Could you check a few things on this model? Use its own coordinates, in mm. Face numbers are marked on the shaded views. A direction names the side the tool comes from. Round coordinates to 2 decimals unless told otherwise and drop trailing zeros. Write each loop counter-clockwise with the first axis right and the second up, starting at its lowest first coordinate (ties: lowest second). Pieces come first, ordered by that corner, then holes. Notation, with made-up numbers: (62, 60.25) - (114, 60.25) arc R17 ccw to (114, 79.25) - close; hole circle Ø7 at (6.5, -9.5). An arc over 180 degrees is marked (long way). Write each question's results on one line, items separated by ' | '. Start each with the question number.
(1) Imagine slicing it at D-D on z = 0.75. Write out the boundary of the cut face in (x, y).
(2) Imagine slicing it at C-C on z = 5. Write out the boundary of the cut face in (x, y).
(3) Imagine slicing it at B-B on y = 3.4. Write out the boundary of the cut face in (x, z).
(4) Imagine slicing it at A-A on x = 8. Write out the boundary of the cut face in (y, z), then the cut area to 3 significant figures.
(5) On a 3-axis mill with a long thin cutter (end or side, diameter ignored), from which of +Z, -Z, +X, -X, +Y, -Y can I reach the whole of each face in a straight line? I mean the marked faces 1, 2 and 3. Say none if no direction works.
(6) For P1, Ø0.9, axis at x = -24, y = 2, coming from the +Z side; P2, Ø2.5, axis at x = -31, y = 1.5, coming from the +Z side; P3, Ø3, axis at y = 2.5, z = 4, coming from the -X side, each with a flat end and sliding along its axis, tell me the tip position at first contact or that it passes through.
(7) Please list where these lines run through material, in increasing order: line 1 (X direction, y = 2, z = 0); line 2 (Z direction, x = 11.5, y = 3.5); line 3 (Y direction, x = -24, z = 3.9). Write a range as [from, to].
```python
from build123d import *

# Parameters (mm, degrees)
SKETCH1_R           = 1.5
BOSS_EXTRUDE1_DEPTH = 5
SKETCH2_W           = 5
SKETCH2_H           = 5
BOSS_EXTRUDE2_DEPTH = 2
SKETCH3_R           = 1.5
CUT_EXTRUDE2_DEPTH  = 3


with BuildPart() as part:
    # Sketch1 → Boss-Extrude1 (new body)
    with BuildSketch(Plane(origin=(0, 0, 0), x_dir=(1, 0, 0), z_dir=(0, 1, 0))):
        with BuildLine():
            Line((-32.5, 4), (32.5, 4))
            ThreePointArc((32.5, 4), (36.5, 0), (32.5, -4))
            Line((32.5, -4), (-32.5, -4))
            ThreePointArc((-32.5, -4), (-36.5, 0), (-32.5, 4))
        make_face()
        with Locations((-32.5, 0)):
            Circle(SKETCH1_R, mode=Mode.SUBTRACT)
        with Locations((32.5, 0)):
            Circle(SKETCH1_R, mode=Mode.SUBTRACT)
        with BuildLine():
            Line((-25, 1.6), (25, 1.6))
            ThreePointArc((25, 1.6), (26.6, 0), (25, -1.6))
            Line((25, -1.6), (-25, -1.6))
            ThreePointArc((-25, -1.6), (-26.6, 0), (-25, 1.6))
        make_face(mode=Mode.SUBTRACT)
    extrude(amount=BOSS_EXTRUDE1_DEPTH)

    # Sketch2 → Boss-Extrude2 (add)
    with BuildSketch(Plane.XY.offset(4)):
        with Locations((-24, 2.5)):
            Rectangle(SKETCH2_W, SKETCH2_H)
    extrude(amount=BOSS_EXTRUDE2_DEPTH)

    # Sketch3 → Cut-Extrude2 (cut)
    with BuildSketch(Plane.XY.offset(6)):
        with Locations((-24, 2.5)):
            Circle(SKETCH3_R)
    extrude(amount=-CUT_EXTRUDE2_DEPTH, mode=Mode.SUBTRACT)


solid = part.part
```
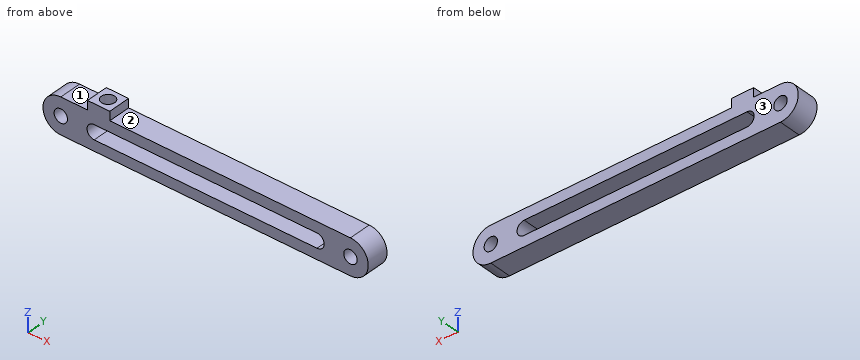
Response:
1) outline: (-36.43, 0) - (-33.8, 0) - (-33.8, 5) - (-36.43, 5) - close; (-31.2, 0) - (-26.41, 0) - (-26.41, 5) - (-31.2, 5) - close; (26.41, 0) - (31.2, 0) - (31.2, 5) - (26.41, 5) - close; (33.8, 0) - (36.43, 0) - (36.43, 5) - (33.8, 5) - close
2) outline: (-26.5, 0) - (-21.5, 0) - (-21.5, 5) - (-26.5, 5) - close; hole circle Ø3 at (-24, 2.5)
3) outline: (-32.5, -4) - (32.5, -4) arc R4 ccw to (32.5, 4) - (-21.5, 4) - (-21.5, 6) - (-22.8, 6) - (-22.8, 3) - (-25.2, 3) - (-25.2, 6) - (-26.5, 6) - (-26.5, 4) - (-32.5, 4) arc R4 ccw to start; hole circle Ø3 at (-32.5, 0); hole (-25, -1.6) - (25, -1.6) arc R1.6 ccw to (25, 1.6) - (-25, 1.6) arc R1.6 ccw to start; hole circle Ø3 at (32.5, 0)
4) outline: (0, -4) - (5, -4) - (5, -1.6) - (0, -1.6) - close; (0, 1.6) - (5, 1.6) - (5, 4) - (0, 4) - close | area: 24.0 mm²
5) face 1: +Z, -X, +Y, -Y | face 2: +Z, +X, +Y, -Y | face 3: +Z, -Z, +X, -X, +Y
6) P1: z = 3 | P2: z = 4 | P3: x = -35.62
7) line 1: [-36.5, -34], [-31, -26.6], [26.6, 31], [34, 36.5] | line 2: [-4, -1.6], [1.6, 4] | line 3: [0, 1], [4, 5]
